from build123d import *

# Parameters (mm, degrees)
BOSS_EXTRUDE1_DEPTH = 4.826
SKETCH3_W           = 441.452
SKETCH3_H           = 63.5
CUT_EXTRUDE1_DEPTH  = 5.826


with BuildPart() as part:
    # Sketch2 → Boss-Extrude1 (new body)
    with BuildSketch(Plane.XY):
        Polygon((0, 122.174), (0, 101.6), (-4.826, 101.6), (-4.826, 76.2), (0, 76.2), (0, 50.8), (-4.826, 50.8), (-4.826, 25.4), (0, 25.4), (0, 0), (431.8, 0), (431.8, 25.4), (436.626, 25.4), (436.626, 50.8), (431.8, 50.8), (431.8, 76.2), (436.626, 76.2), (436.626, 101.6), (431.8, 101.6), (431.8, 122.174), (406.4, 122.174), (406.4, 127), (381, 127), (381, 122.174), (355.6, 122.174), (355.6, 127), (330.2, 127), (330.2, 122.174), (304.8, 122.174), (304.8, 127), (279.4, 127), (279.4, 122.174), (254, 122.174), (254, 127), (228.6, 127), (228.6, 122.174), (203.2, 122.174), (203.2, 127), (177.8, 127), (177.8, 122.174), (152.4, 122.174), (152.4, 127), (127, 127), (127, 122.174), (101.6, 122.174), (101.6, 127), (76.2, 127), (76.2, 122.174), (50.8, 122.174), (50.8, 127), (25.4, 127), (25.4, 122.174), align=None)
    extrude(amount=BOSS_EXTRUDE1_DEPTH)

    # Sketch3 → Cut-Extrude1 (cut, through all)
    with BuildSketch(Plane(origin=(0, 0, 0), x_dir=(-1, 0, 0), z_dir=(0, 0, -1))):
        with Locations((-215.9, 31.75)):
            Rectangle(SKETCH3_W, SKETCH3_H)
    extrude(amount=-CUT_EXTRUDE1_DEPTH, mode=Mode.SUBTRACT)


solid = part.part
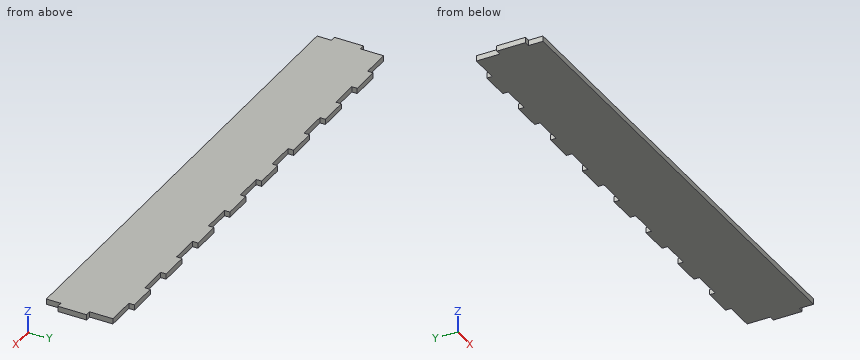
Geometry: final body of the model. Coordinates: model frame, mm. Give positions to 0.01 mm unless a question says otherwise; leave off trailing zeros. Write each loop counter-clockwise with the first axis right and the second up, starting at its lowest first coordinate (ties: lowest second). Pieces come first, ordered by that corner, then holes.
(1) First-contact query: P1, Ø2.5, axis at y = 125, z = 2.5, coming from the +X side; P2, Ø1.4, axis at y = 109, z = 3, coming from the +X side; P3, Ø1.4, axis at y = 125, z = 2, coming from the -X side. Flat tips, straight axial feed; report the tip coordinate or a pass-through.
(2) Cut plane A-A, the plane x = 63. Return loops of the section in (y, z), then the cut area to 3 significant figures.
(3) Ray query, line 1 (Y direction, x = 102.5, z = 2.15); line 2 (X direction, y = 66.5, z = 1.95). Return the intervals inside material, ascending.
(4) Cut plane B-B, the plane y = 117.5. Return loops of the section in (x, z), then the cut area to 3 significant figures.
Values follow:
1. P1: stops at x = 406.4
1. P2: stops at x = 431.8
1. P3: stops at x = 25.4
2. outline: (63.5, 0) - (122.17, 0) - (122.17, 4.83) - (63.5, 4.83) - close
2. area: 283 mm2
3. line 1: y = 63.5 to 122.17
3. line 2: x = 0 to 431.8
4. outline: (0, 0) - (431.8, 0) - (431.8, 4.83) - (0, 4.83) - close
4. area: 2,080 mm2
